Drawing for the job (mm, zero at the part's lowest x, y, z). A direction names the side the tool comes from. Round coordinates to 2 decimals unless told otherwise and drop trailing zeros. Write each loop counter-clockwise with the first axis right and the second up, starting at its lowest first coordinate (ties: lowest second). Pieces come first, ordered by that corner, then holes. Notation, with made-up numbers: (8, 18) -> (36, 18) arc R34 cw to (36, 53) -> close; hole circle Ø4 at (45.5, -6). An arc over 180 degrees is marked (long way). Answer in a Markdown table with one row per item. Add a question column.
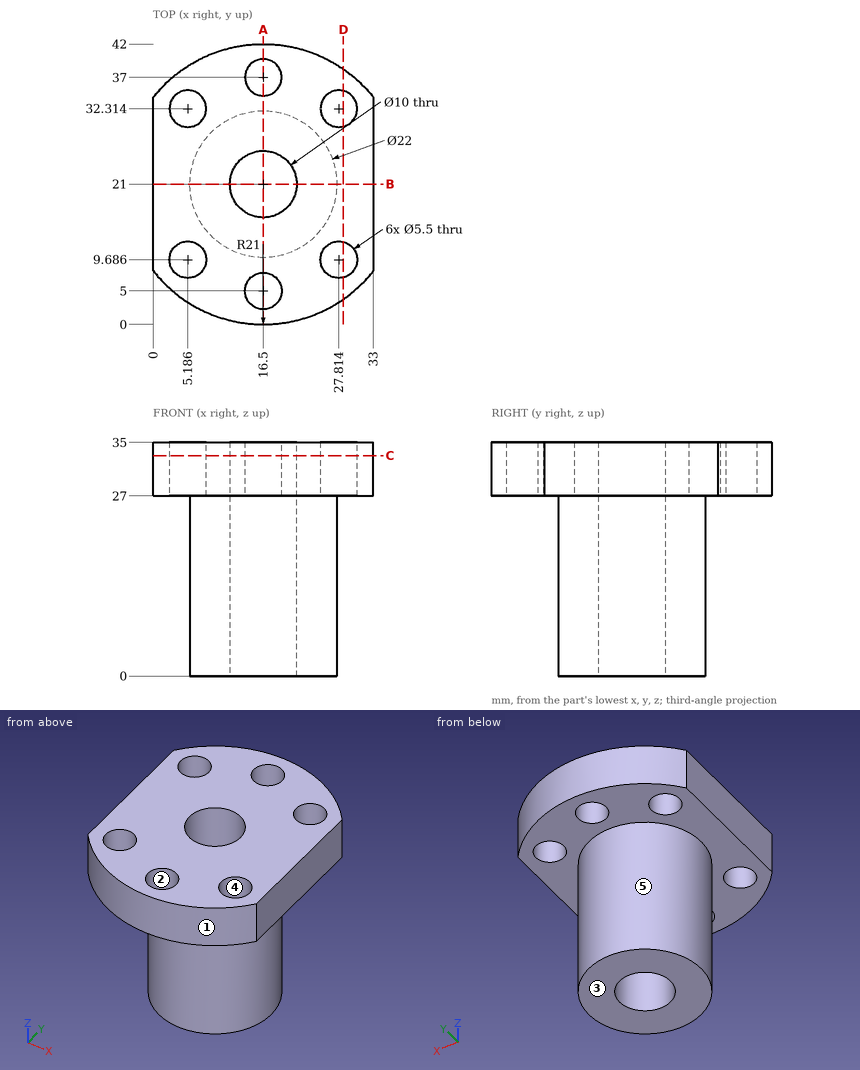
(1) Drop flat-ended pins along their axis: P1, Ø7, axis at x = 16.5, y = 5, coming from the -Z side; P2, Ø2, axis at y = 12.5, z = 5.5, coming from the +X side; P3, Ø12, axis at x = 12.5, z = 22, coming from the -Y side. Give the stop position or say it passes through.
(2) Mould opens along X. For the marked faces 1, 2 and 3 say: pulls with the +X half, pulls with the -X half, needs draft (parallel to the pull), parting line crosses it, or undercut.
(3) Saw through at C-C (z = 33). List the corners of the cut face in (x, y), plus the area to 3 significant figures.
(4) Which spindle directions (+Z, -Z, +X, -X, +Y, -Y) get a long thin tool onto all of the face, cutting with end or side? Do the marked faces 4 and 5. Say none if no direction does.
(5) Probe line 1 along Y through (x, z) = (17.5, 29); line 2 along Z through (x, y) = (30.5, 11); line 3 along X through (y, z) = (35.5, 33.5) (1 decimal). List the from-to ranges inside material, lowest first.
(6) Saw through at B-B (y = 21). List the corners of the cut face in (x, z), plus the area to 3 significant figures.
(7) Saw through at A-A (x = 16.5). List the corners of the cut face in (y, z), plus the area to 3 significant figures.
(8) Saw through at D-D (x = 28.5). List the corners of the cut face in (y, z).
Answer sheet:
| question | item | result |
|---|---|---|
| 1 | P1 | stops at z = 27 |
| 1 | P2 | stops at x = 24.55 |
| 1 | P3 | stops at y = 0.01 |
| 2 | face 1 | parting line crosses it |
| 2 | face 2 | undercut |
| 2 | face 3 | needs draft |
| 3 | outline | (0, 8.01) arc R21 ccw to (33, 8.01) -> (33, 33.99) arc R21 ccw to (0, 33.99) -> close; hole circle Ø5.5 at (5.19, 9.69); hole circle Ø5.5 at (5.19, 32.31); hole circle Ø10 at (16.5, 21); hole circle Ø5.5 at (16.5, 5); hole circle Ø5.5 at (16.5, 37); hole circle Ø5.5 at (27.81, 9.69); hole circle Ø5.5 at (27.81, 32.31) |
| 3 | area | 1,000 mm² |
| 4 | face 4 | +Z, -Z |
| 4 | face 5 | -Z |
| 5 | line 1 | y = 0.02 to 2.44, 7.56 to 16.1, 25.9 to 34.44, 39.56 to 41.98 |
| 5 | line 2 | z = 27 to 35 |
| 5 | line 3 | x = 1.3 to 14.2, 18.8 to 31.7 |
| 6 | outline | (0, 27) -> (5.5, 27) -> (5.5, 0) -> (11.5, 0) -> (11.5, 35) -> (0, 35) -> close; (21.5, 0) -> (27.5, 0) -> (27.5, 27) -> (33, 27) -> (33, 35) -> (21.5, 35) -> close |
| 6 | area | 508 mm² |
| 7 | outline | (0, 27) -> (2.25, 27) -> (2.25, 35) -> (0, 35) -> close; (7.75, 27) -> (10, 27) -> (10, 0) -> (16, 0) -> (16, 35) -> (7.75, 35) -> close; (26, 0) -> (32, 0) -> (32, 27) -> (34.25, 27) -> (34.25, 35) -> (26, 35) -> close; (39.75, 27) -> (42, 27) -> (42, 35) -> (39.75, 35) -> close |
| 7 | area | 492 mm² |
| 8 | outline | (3.77, 27) -> (7.02, 27) -> (7.02, 35) -> (3.77, 35) -> close; (12.35, 27) -> (29.65, 27) -> (29.65, 35) -> (12.35, 35) -> close; (34.98, 27) -> (38.23, 27) -> (38.23, 35) -> (34.98, 35) -> close |
